Source: CAD feature listing. Evaluate the final solid. Frame: model axes, mm. Round coordinates to 2 decimals unless told otherwise and drop trailing zeros. Write each loop counter-clockwise with the first axis right and the second up, starting at its lowest first coordinate (ties: lowest second). Pieces come first, ordered by that corner, then holes. Notation, with made-up numbers: M 86.25,83.5 L 130.25,83.5 A15 ccw 130.25,102.5 Z; hole C 44.25,-24.75 d9. An arc over 180 degrees is marked long. Answer in a Markdown table with one row per item.
from build123d import *

# Parameters (mm, degrees)
F0_R     = 4
F0_R_2   = 1.5
F0_R_3   = 2.5
F0_R_4   = 2
F1_DEPTH = 0.5
F2_SIZE  = 4


with BuildPart() as f1:
    # F0 (on Top) → F1 (new body, symmetric)
    with BuildSketch(Plane.XY):
        Polygon((-92.5, 127.5), (-92.5, 0), (-92.5, -127.5), (-60, -127.5), (-60, -142.5), (0, -142.5), (60, -142.5), (60, -127.5), (92.5, -127.5), (92.5, 0), (92.5, 127.5), (60, 127.5), (60, 142.5), (0, 142.5), (-60, 142.5), (-60, 127.5), align=None)
        with Locations((-84.5, -120)):
            Circle(F0_R, mode=Mode.SUBTRACT)
        with Locations((-63, -61.5)):
            Circle(F0_R_2, mode=Mode.SUBTRACT)
        with Locations((-32.5, -2.5)):
            Circle(F0_R_3, mode=Mode.SUBTRACT)
        with Locations((48, -130)):
            Circle(F0_R_4, mode=Mode.SUBTRACT)
        with Locations((84.5, -120)):
            Circle(F0_R, mode=Mode.SUBTRACT)
        with Locations((27.5, -2.5)):
            Circle(F0_R_3, mode=Mode.SUBTRACT)
        with Locations((63, -61.5)):
            Circle(F0_R_2, mode=Mode.SUBTRACT)
        with Locations((-85, 12.5)):
            Circle(F0_R_3, mode=Mode.SUBTRACT)
        with Locations((-63, 61.5)):
            Circle(F0_R_2, mode=Mode.SUBTRACT)
        with Locations((-84.5, 120)):
            Circle(F0_R, mode=Mode.SUBTRACT)
        with Locations((-7.5, 102.5)):
            Circle(F0_R_3, mode=Mode.SUBTRACT)
        with Locations((85, 12.5)):
            Circle(F0_R_3, mode=Mode.SUBTRACT)
        with Locations((63, 61.5)):
            Circle(F0_R_2, mode=Mode.SUBTRACT)
        with Locations((32.5, 102.5)):
            Circle(F0_R_3, mode=Mode.SUBTRACT)
        with Locations((84.5, 120)):
            Circle(F0_R, mode=Mode.SUBTRACT)
    extrude(amount=F1_DEPTH, both=True)

    # F2
    f2_edges = [f1.edges().sort_by_distance(p)[0] for p in [
        (-92.5, 127.5, 0),
        (-60, 142.5, 0),
        (60, 142.5, 0),
        (92.5, 127.5, 0),
        (92.5, -127.5, 0),
        (60, -142.5, 0),
        (-60, -142.5, 0),
        (-92.5, -127.5, 0),
    ]]
    chamfer(f2_edges, length=F2_SIZE)


solid = f1.part
Q1. Section A-A (y = 120). Return loops of the section in (x, z), and give its area (3 significant figures).
Solutions:
| item | result |
|---|---|
| outline | M -92.5,-0.5 L -88.5,-0.5 L -88.5,0.5 L -92.5,0.5 Z; M -80.5,-0.5 L 80.5,-0.5 L 80.5,0.5 L -80.5,0.5 Z; M 88.5,-0.5 L 92.5,-0.5 L 92.5,0.5 L 88.5,0.5 Z |
| area | 169 mm2 |
Q2. Contact query for a flat-ended pin moving along its axis: pin 1 Ø0.5 at (x, z) = (-69.5, 0) entering from -Y. Output: stop coordinate, or through.
Solutions:
| item | result |
|---|---|
| pin 1 | stops at y = -127.5 |
Q3. Section B-B (z = 0). State how many separate pieces and enclosed holes the cut face has, and give its area (3 significant figures).
Solutions:
| item | result |
|---|---|
| separate pieces | 1 |
| enclosed holes | 15 |
| area | 50,400 mm2 |
Q4. Section C-C (x = 76.5). Return loops of the section in (y, z), and give its area (3 significant figures).
Solutions:
| item | result |
|---|---|
| outline | M -127.5,-0.5 L 127.5,-0.5 L 127.5,0.5 L -127.5,0.5 Z |
| area | 255 mm2 |
Q5. Material intervals for probe 1 along Y at (x, z) = (-63, 0.1); probe 2 along Y at (x, z) = (48, 0.1); probe 3 along Y at (x, z) = (-32.5, 0.25), sorted ascending.
Solutions:
| item | result |
|---|---|
| probe 1 | y = -127.5 to -63, -60 to 60, 63 to 127.5 |
| probe 2 | y = -142.5 to -132, -128 to 142.5 |
| probe 3 | y = -142.5 to -5, 0 to 142.5 |
Q6. Pull-direction query (X, two-part tool) for faces 1 (the cylindrical face through (83.979, -116.034, -0.007)), 2 (the flat face through (-1, 2, 0.5)); classes: pulls with the +X half, pulls with the -X half, needs draft (parallel to the pull), parting line crosses it, or undercut.
Solutions:
| item | result |
|---|---|
| face 1 | undercut |
| face 2 | needs draft |
